Build history of the part. All positions in model axes, mm. A direction names the side the tool comes from. Round coordinates to 2 decimals unless told otherwise and drop trailing zeros. Write each loop counter-clockwise with the first axis right and the second up, starting at its lowest first coordinate (ties: lowest second). Pieces come first, ordered by that corner, then holes. Notation, with made-up numbers: (25.5, 8) -> (67.5, 8) arc R17 cw to (67.5, 33) -> close; hole circle Ø10 at (11.25, 45.5). An arc over 180 degrees is marked (long way). Return JSON: item names as keys, results as strings.
from build123d import *

# Parameters (mm, degrees)
F0_R     = 8
F1_DEPTH = 15.8
F2_R     = 8
F2_R_2   = 5
F3_DEPTH = 7.8
F4_R     = 3.1
F5_DEPTH = 25
F6_SIZE  = 0.5


with BuildPart() as f1:
    # F0 (on Right) → F1 (new body)
    with BuildSketch(Plane.YZ):
        Circle(F0_R)
    extrude(amount=-F1_DEPTH)

    # F2 (on face) → F3 (cut)
    with BuildSketch(Plane.YZ):
        Circle(F2_R)
        Circle(F2_R_2, mode=Mode.SUBTRACT)
    extrude(amount=-F3_DEPTH, mode=Mode.SUBTRACT)

    # F4 (on face) → F5 (cut)
    with BuildSketch(Plane.YZ):
        Circle(F4_R)
    extrude(amount=-F5_DEPTH, mode=Mode.SUBTRACT)

    # F6
    f6_edges = [f1.edges().sort_by_distance(p)[0] for p in [
        (0, -3.1, 0),
        (-15.8, -3.1, 0),
        (0, -5, 0),
        (-7.8, -5, 0),
        (-7.8, -8, 0),
        (-15.8, -8, 0),
    ]]
    chamfer(f6_edges, length=F6_SIZE)


solid = f1.part
Q1. Saw through at A-A on y = 0. List the corners of the cut face in (x, z).
Verdict:
{"outline": "(-15.8, -7.5) -> (-15.3, -8) -> (-8.3, -8) -> (-7.8, -7.5) -> (-7.8, -5.5) -> (-7.3, -5) -> (-0.5, -5) -> (0, -4.5) -> (0, -3.6) -> (-0.5, -3.1) -> (-15.3, -3.1) -> (-15.8, -3.6) -> close; (-15.8, 3.6) -> (-15.3, 3.1) -> (-0.5, 3.1) -> (0, 3.6) -> (0, 4.5) -> (-0.5, 5) -> (-7.3, 5) -> (-7.8, 5.5) -> (-7.8, 7.5) -> (-8.3, 8) -> (-15.3, 8) -> (-15.8, 7.5) -> close"}
Q2. Saw through at C-C on x = -1.25. List the corners of the cut face in (y, z), then the cut area to 3 significant figures.
Verdict:
{"outline": "circle Ø10 at (0, 0); hole circle Ø6.2 at (0, 0)", "area": "48.3 mm²"}
Q3. Two-plate mould, pull along Z, no slides. Class faces 3 (the cylindrical face through (-11.75, -1.73, -7.81)), 4 (the cylindrical face through (-7.8, 1.43, -2.75)), 5 (the flat face through (-15.8, 1.6, 3.4)): +Z half, -Z half, draft (parallel to the pull), parting line (faces both ways), or undercut.
Verdict:
{"face 3": "parting line", "face 4": "undercut", "face 5": "draft"}
Q4. 3-axis set-ups, long thin cutter, end or side, ignore diameter. For faces 1 (the cylindrical face through (-3.85, -1.08, -4.88)), 2 (the flat face through (0, 0, 4)): which of +Z, -Z, +X, -X, +Y, -Y reach the whole face in a straight line?
Verdict:
{"face 1": "+X", "face 2": "+Z, -Z, +X, +Y, -Y"}
Q5. Wall check: L1, parallel to Z at x = -6.25, y = 0; L2, parallel to X at y = -6.75, z = 0.25; L3, parallel to Y at x = -13.25, z = -2. Give the ranges that are in metal, low to high.
Verdict:
{"L1": "z = -5 to -3.1, 3.1 to 5", "L2": "x = -15.8 to -7.8", "L3": "y = -7.75 to -2.37, 2.37 to 7.75"}
Q6. Saw through at D-D on x = -13.25. List the corners of the cut face in (y, z), then the cut area to 3 significant figures.
Verdict:
{"outline": "circle Ø16 at (0, 0); hole circle Ø6.2 at (0, 0)", "area": "171 mm²"}
Q7. Pin check, flat tips, straight feed: pin 1 Ø3 at (x, y) = (-2, -6) entering from -Z; pin 2 Ø3 at (x, z) = (-13.5, 6) entering from -Y; pin 3 Ø1.5 at (x, z) = (-10.5, 5.5) entering from -Y. Stop position of each tip, or through.
Verdict:
{"pin 1": "stops at z = -2.18", "pin 2": "stops at y = -6.61", "pin 3": "stops at y = -6.44"}
